Input: part model. Units: mm. Frame: model coordinates. A direction names the side the tool comes from. Give positions to 0.01 mm unless a question says otherwise; leave off trailing zeros. Write each loop counter-clockwise with the first axis right and the second up, starting at its lowest first coordinate (ties: lowest second). Pieces come first, ordered by that corner, then holes. Notation, with made-up numbers: (-15, -24.5) - (21, -24.5) arc R4 cw to (21, -19.5) - close; hole circle Ø2 at (42.5, 64). An arc over 180 degrees is marked (long way). Answer as CSV lines item,"result".
```python
from build123d import *

# Parameters (mm, degrees)
F0_W     = 9.525
F0_H     = 15.875
F0_R     = 1.905
F1_DEPTH = 3.175
F0_H_2   = 3.175
F2_DEPTH = 12.7
F3_R     = 1.905
F4_DEPTH = 25.4


with BuildPart() as f1:
    # F0 (on Top) → F1 (new body)
    with BuildSketch(Plane.XY):
        with Locations((0, 1.5875)):
            Rectangle(F0_W, F0_H)
        with Locations((0, 5.715)):
            Circle(F0_R, mode=Mode.SUBTRACT)
    extrude(amount=F1_DEPTH)

    # F0 (on Top) → F2 (join)
    with BuildSketch(Plane.XY):
        with Locations((0, -7.9375)):
            Rectangle(F0_W, F0_H_2)
    extrude(amount=F2_DEPTH)

    # F3 (on face) → F4 (cut)
    with BuildSketch(Plane(origin=(0, -6.35, 0), x_dir=(-1, 0, 0), z_dir=(0, 1, 0))):
        with Locations((0, 7.9375)):
            Circle(F3_R)
    extrude(amount=-F4_DEPTH, mode=Mode.SUBTRACT)


solid = f1.part
```
Item 1: Mould query, pull axis Z, two halves, no side actions, for faces 1 (the face through (0.248, -7.915, 9.826)), 2 (the face through (0, -8, 12.7)), 3 (the face through (-4.762, -4, 2)). Classes: +Z half, -Z half, draft (parallel to the pull), parting line (faces both ways), or undercut.
The answers:
face 1,"undercut"
face 2,"+Z half"
face 3,"draft"
Item 2: Cut plane D-D on x = -1.5. Return the cut outline in (y, z) (3 decimals).
The answers:
outline,"(-9.525, 0) - (4.541, 0) - (4.541, 3.175) - (-6.35, 3.175) - (-6.35, 6.763) - (-9.525, 6.763) - close; (-9.525, 9.112) - (-6.35, 9.112) - (-6.35, 12.7) - (-9.525, 12.7) - close; (6.889, 0) - (9.525, 0) - (9.525, 3.175) - (6.889, 3.175) - close"
Item 3: Cut plane B-B on z = 1. Return the cut outline in (x, y) (1 decimal).
The answers:
outline,"(-4.8, -9.5) - (4.8, -9.5) - (4.8, 9.5) - (-4.8, 9.5) - close; hole circle Ø3.8 at (0, 5.7)"
Item 4: Contact query for flat-ended pins moving along their axis: pin 1 (4.5 mm diameter, centred on x = 0, z = 7.94, fed in from -Y) (3 decimals); pin 2 (3 mm diameter, centred on x = -1.5, y = -0.5, fed in from +Z) (3 decimals); pin 3 (5 mm diameter, centred on x = -0.5, z = 10, fed in from +Y); pin 4 (1 mm diameter, centred on y = -4.5, z = 10, fed in from -X). Output: stop coordinate, or through.
The answers:
pin 1,"y = -9.525"
pin 2,"z = 3.175"
pin 3,"y = -6.35"
pin 4,"through"
Item 5: Cut plane A-A on x = 0. Count the separate pieces of the cut face and the enclosed holes in it, plus the area to 3 significant figures.
The answers:
separate pieces,"3"
enclosed holes,"0"
area,"66.5 mm²"
Item 6: Cut plane C-C on y = -0.75. Return the cut outline in (x, z) (1 decimal).
The answers:
outline,"(-4.8, 0) - (4.8, 0) - (4.8, 3.2) - (-4.8, 3.2) - close"
Item 7: Ray query, line 1 (Y direction, x = 0, z = 1.75) (3 decimals); line 2 (Z direction, x = 0, y = -8.6); line 3 (Z direction, x = 3, y = -1.25) (3 decimals). Return the intervals inside material, ascending. Write a range as from..to.
The answers:
line 1,"-9.525..3.81, 7.62..9.525"
line 2,"0..6.03, 9.84..12.7"
line 3,"0..3.175"
Item 8: Reachability of faces 4 (the face through (0, 9.525, 2)), 5 (the face through (-0.1, -6.35, 5.8)) from +Z, -Z, +X, -X, +Y, -Y: full face, straight path, thin tool, end or side. Return the list, or none.
The answers:
face 4,"+Z, -Z, +X, -X, +Y"
face 5,"+Z, +X, -X, +Y"
